The model under review builds one solid part; all positions refer to its coordinate system, in mm. Face numbers are marked on the shaded views. A direction names the side the tool comes from. Coordinates: 2 decimals unless noted, no trailing zeros. Order: outer loops, then holes, each group sorted by start corner. A loop starts at its lowest first (then second) coordinate and runs counter-clockwise, first axis right, second up. Notation, with made-up numbers: (-1.5, 30) - (37.5, 30) arc R33 ccw to (37.5, 64) - close; hole circle Ø9 at (51.25, 15). An arc over 180 degrees is marked (long way). Answer in a Markdown table with one row per item.
```python
from build123d import *

# Parameters (mm, degrees)
SKETCH2_R           = 2
BOSS_EXTRUDE2_DEPTH = 80
CHAMFER2_SIZE       = 5
CUT_EXTRUDE1_REACH  = 133.355
SKETCH3_R           = 3.5


with BuildPart() as part:
    # Sketch2 → Boss-Extrude2 (new body)
    with BuildSketch(Plane(origin=(0, 0, 0), x_dir=(0, 0, -1), z_dir=(1, 0, 0))):
        Polygon((89.086021447, -37.960779863), (77.429167198, -49.617634112), (-24.612463363, -49.617634112), (-36.269317612, -37.960779863), (-36.269317612, 24.080850698), (-24.612463363, 35.737704947), (35.760119639, 35.737704947), (35.760119639, 29.578296595), (50.725478568, 26.014986706), (52.846798911, 28.136307049), (45.245401014, 35.737704947), (53.377128997, 35.737704947), (55.675226036, 38.035801986), (54.973323075, 38.737704947), (-39.269317612, 38.737704947), (-39.269317612, -52.617634112), (92.086021447, -52.617634112), (92.086021447, 1.625006575), (91.384118486, 2.326909536), (89.086021447, 0.028812497), (89.086021447, -8.102915487), (81.484279552, -0.501173592), (79.362959209, -2.622493935), (79.363303206, -2.622837932), (82.926613095, -17.588196861), (89.086021447, -17.588196861), align=None)
        with Locations((86.086021447, -46.617634112)):
            Circle(SKETCH2_R, mode=Mode.SUBTRACT)
        with Locations((-33.269317612, -46.617634112)):
            Circle(SKETCH2_R, mode=Mode.SUBTRACT)
        with Locations((86.086021447, -13.588196861)):
            Circle(SKETCH2_R, mode=Mode.SUBTRACT)
        with Locations((-33.269317612, 32.737704947)):
            Circle(SKETCH2_R, mode=Mode.SUBTRACT)
        with Locations((39.760119639, 32.737704947)):
            Circle(SKETCH2_R, mode=Mode.SUBTRACT)
    extrude(amount=BOSS_EXTRUDE2_DEPTH)

    # Chamfer2
    chamfer2_edges = [part.edges().sort_by_distance(p)[0] for p in [
        (40, -52.617634112, -92.086021447),
        (40, -52.617634112, 39.269317612),
        (40, 38.737704947, 39.269317612),
    ]]
    chamfer(chamfer2_edges, length=CHAMFER2_SIZE)

    # Sketch3 → Cut-Extrude1 (cut, up to next)
    with BuildSketch(Plane(origin=(0, 0, -92.086021447), x_dir=(-1, 0, 0), z_dir=(0, 0, -1)), mode=Mode.PRIVATE) as cut_extrude1_sk1:
        with Locations((-40, -27.617634112)):
            Circle(SKETCH3_R)
    cut_extrude1_tool1 = extrude(cut_extrude1_sk1.sketch, amount=-CUT_EXTRUDE1_REACH, mode=Mode.PRIVATE) & part.part
    add(cut_extrude1_tool1.solids().sort_by_distance((40, -27.617634, -92.086021))[0], mode=Mode.SUBTRACT)


solid = part.part
```
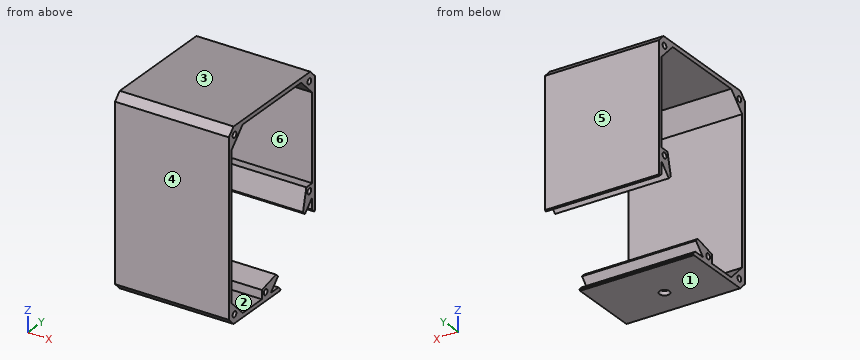
Item 1: We need section A-A, the plane z = -12. Write out the cut boundary in (x, y), then the cut area to 3 significant figures.
Check values:
| item | result |
|---|---|
| outline | (0, -52.62) - (80, -52.62) - (80, -49.62) - (0, -49.62) - close; (0, 35.74) - (80, 35.74) - (80, 38.74) - (0, 38.74) - close |
| area | 480 mm^2 |
Item 2: We need section B-B, the plane y = -29.5. Write out the cut boundary in (x, z), then the cut area to 3 significant figures.
Check values:
| item | result |
|---|---|
| outline | (0, -92.09) - (37.05, -92.09) - (37.05, -89.09) - (0, -89.09) - close; (0, 36.27) - (80, 36.27) - (80, 39.27) - (0, 39.27) - close; (42.95, -92.09) - (80, -92.09) - (80, -89.09) - (42.95, -89.09) - close |
| area | 462 mm^2 |
Item 3: To check wall thickness, follow line 1 (Y direction, x = 42, z = -21.5); line 2 (Z direction, x = 68, y = -28); line 3 (Z direction, x = 20.5, y = -7). State the ranges of each line that lie inside material, in increasing order. Write a range as from..to.
Check values:
| item | result |
|---|---|
| line 1 | -52.62..-49.62, 35.74..38.74 |
| line 2 | -92.09..-89.09, 36.27..39.27 |
| line 3 | -92.09..-89.09, -87.98..-80.41, 36.27..39.27 |
Item 4: Mouldability with a two-part tool opening along Y and no side actions: class the marked faces 3, 4, 5 and 6 as +Y half, -Y half, draft (parallel to the pull), parting line (faces both ways), or undercut.
Check values:
| item | result |
|---|---|
| face 3 | draft |
| face 4 | -Y half |
| face 5 | +Y half |
| face 6 | undercut |
Item 5: Tool access review of the marked faces 1 and 2: name each direction out of +Z, -Z, +X, -X, +Y, -Y from which nothing blocks a thin tool from reaching the whole face with its end or side.
Check values:
| item | result |
|---|---|
| face 1 | -Z, +X, -X, +Y, -Y |
| face 2 | +X, -X |
Item 6: Clearance check with flat-ended pins moving along their axes: pin 1 Ø5 at (y, z) = (-46.62, -86.09) entering from -X; pin 2 Ø4 at (x, y) = (40, -27.62) entering from -Z; pin 3 Ø3 at (x, z) = (8.5, -72.5) entering from +Y; pin 4 Ø2.5 at (y, z) = (32.74, 33.27) entering from +X (3 decimals). State where each tip first meets the part, or that it passes through.
Check values:
| item | result |
|---|---|
| pin 1 | x = 0 |
| pin 2 | z = 36.27 |
| pin 3 | y = -49.62 |
| pin 4 | through |
Item 7: We need section C-C, the plane x = 74. State how many separate pieces and enclosed holes the cut face has, then the cut area to 3 significant figures.
Check values:
| item | result |
|---|---|
| separate pieces | 1 |
| enclosed holes | 5 |
| area | 1,410 mm^2 |
